```python
from build123d import *

# Parameters (mm, degrees)
F0_W     = 150
F0_H     = 150
F1_DEPTH = 20
F2_R     = 5
F3_DEPTH = 20.001
F4_SIZE  = 5


with BuildPart() as f1:
    # F0 (on Front) → F1 (new body)
    with BuildSketch(Plane.XZ):
        Rectangle(F0_W, F0_H)
    extrude(amount=F1_DEPTH)

    # F2 (on face) → F3 (cut, through all)
    with BuildSketch(Plane.XZ.offset(20)):
        with Locations((0, -45)):
            Circle(F2_R)
    extrude(amount=-F3_DEPTH, mode=Mode.SUBTRACT)

    # F4
    f4_edges = [f1.edges().sort_by_distance(p)[0] for p in [
        (75, -10, 75),
        (-75, -10, 75),
        (0, 0, 75),
        (0, -20, 75),
        (75, -10, -75),
        (75, 0, 0),
        (75, -20, 0),
        (-75, -10, -75),
        (0, 0, -75),
        (0, -20, -75),
        (-75, 0, 0),
        (-75, -20, 0),
    ]]
    chamfer(f4_edges, length=F4_SIZE)


solid = f1.part
```
The listing builds one solid part. Answer for the finished solid, in the listing's coordinates (mm). Give positions to 0.01 mm unless a question says otherwise; leave off trailing zeros. Order: outer loops, then holes, each group sorted by start corner. A loop starts at its lowest first (then second) coordinate and runs counter-clockwise, first axis right, second up. Notation, with made-up numbers: M 82.25,-25 L 124.25,-25 A15 ccw 124.25,-12 Z; hole C 5,53 d2. An arc over 180 degrees is marked long. Put each result on its own line as item: value. Start each with the question number.
Item 1: The part is cut by section D-D, the plane z = -2. Determine the outline of the cut face in (x, y), and give its area (3 significant figures).
Item 2: Find the intervals of material crossed by line 1 along Z through (x, y) = (0, -6); line 2 along Z through (x, y) = (0, -4.5); line 3 along Z through (x, y) = (-65, -3), in increasing order.
Item 3: Flat-ended cylindrical pins translate along their axes: P1, Ø3, axis at x = 10.5, y = -17, coming from the +Z side; P2, Ø11.5, axis at x = 0, z = -45, coming from the +Y side. Find the tip coordinate at first contact, or state that the pin passes through.
Item 4: The part is cut by section B-B, the plane z = -45. Determine the outline of the cut face in (x, y).
Item 5: For a pull along Z with two mould halves and no side action, classify faces 1 (the face through (73, -10, 72)), 2 (the face through (-1, -2, -72)), 3 (the face through (73, -17, -1)) as +Z half, -Z half, draft (parallel to the pull), parting line (faces both ways), or undercut.
Item 6: The part is cut by section A-A, the plane x = 0. Determine the outline of the cut face in (y, z), and give its area (3 significant figures).
Item 7: The part is cut by section C-C, the plane y = -17.5. Determine the outline of the cut face in (x, z), and give its area (3 significant figures).
Answer key:
1. outline: M -75,-15 L -70,-20 L 70,-20 L 75,-15 L 75,-5 L 70,0 L -70,0 L -75,-5 Z
1. area: 2,950 mm²
2. line 1: z = -75 to -50, -40 to 75
2. line 2: z = -74.5 to -50, -40 to 74.5
2. line 3: z = -73 to 73
3. P1: stops at z = 74.5
3. P2: stops at y = 0
4. outline: M -75,-15 L -70,-20 L -5,-20 L -5,0 L -70,0 L -75,-5 Z; M 5,-20 L 70,-20 L 75,-15 L 75,-5 L 70,0 L 5,0 Z
5. face 1: +Z half
5. face 2: -Z half
5. face 3: draft
6. outline: M -20,-70 L -15,-75 L -5,-75 L 0,-70 L 0,-50 L -20,-50 Z; M -20,-40 L 0,-40 L 0,70 L -5,75 L -15,75 L -20,70 Z
6. area: 2,750 mm²
7. outline: M -72.5,-70 L -70,-72.5 L 70,-72.5 L 72.5,-70 L 72.5,70 L 70,72.5 L -70,72.5 L -72.5,70 Z; hole C 0,-45 d10
7. area: 20,900 mm²
